Autodesk Inventor part; units mm, degrees
ref_plane "Plano de trabajo4" through (10, 0, 0) normal (1, 0, 0) x (0, 1, 0)
ref_plane "YZ Plane" through (0, 0, 0) normal (1, 0, 0) x (0, 1, 0)
ref_plane "XZ Plane" through (0, 0, 0) normal (0, 1, 0) x (-1, 0, 0)
sketch "Boceto1" plane through (0, 0, 0) normal (0, 0, 1) x (1, 0, 0)
  line L0 (0, 0) -> (20, 0)
  line L1 (20, 0) -> (20, 18.75)
  line L2 (20, 18.75) -> (0, 18.75)
  line L3 (0, 18.75) -> (0, 0)
  point P0 (9.375, 9.375)
  dimension "d0" = 20
  dimension "d10" = 18.75
extrude "Extrusión1" add sketch "Boceto1" against normal blind 56.25
sketch "Boceto2" plane through (0, 0, 0) normal (0, 0, 1) x (1, 0, 0)
  circle A0 centre (10, 9.375) radius 4
  line L0 (0, 0) -> (20, 0)
  line L1 (0, 18.75) -> (0, 0)
  point P0 (10, 0)
  point P1 (0, 9.375)
  dimension "d3" = 8
extrude "Extrusión2" cut sketch "Boceto2" against normal blind 10
fillet "Empalme1" radius 2 4 edges at (20, 0, -28.125) (0, 0, -28.125) (0, 18.75, -28.125) (20, 18.75, -28.125)
sketch "Boceto3" plane through (0, 0, -56.25) normal (0, 0, -1) x (-1, 0, 0)
  line L0 (-20, 16.75) -> (-20, 2)
  line L1 (-18, 0) -> (-2, 0)
  line L2 (-5, 18.75) -> (-15, 18.75)
  line L3 (-15, 18.75) -> (-15, 0)
  line L4 (-15, 0) -> (-5, 0)
  line L5 (-5, 0) -> (-5, 18.75)
  line L6 (-5, 18.75) -> (-15, 0) construction
  line L7 (-15, 18.75) -> (-5, 0) construction
  line L8 (-2, 18.75) -> (-18, 18.75)
  point P0 (0, 0)
  point P1 (-10, 10)
  point P2 (-10, 9.375)
  dimension "d11" = 10
extrude "Extrusión3" cut sketch "Boceto3" against normal blind 10
ref_plane "Plano de trabajo4" through (10, 0, 0) normal (1, 0, 0) x (0, 1, 0)
sketch "Boceto5" plane through (0, 2, 0) normal (-1, 0, 0) x (0, 0, 1)
  circle A0 centre (-28.125, 7) radius 4
  line L0 (0, 14.75) -> (0, 0)
  line L1 (0, 0) -> (-56.25, 0)
  point P0 (0, -2)
  dimension "d20" = 8
  dimension "d21" = 28.125
  dimension "d22" = 7
extrude "Extrusión5" add sketch "Boceto5" along normal blind 10 and the other way blind 30
sketch "Boceto6" plane through (15, 0, -56.25) normal (-1, 0, 0) x (0, 0, 1)
  line L0 (0, 0) -> (56.25, 0)
  line L1 (56.25, 13.375) -> (56.25, 5.375)
  arc A0 (2.5, 12.4975) -> (7.5, 12.4975) centre (5, 9.375) ccw
  line L2 (2.5, 12.4975) -> (7.5, 12.4975)
  line L3 (7.5, 12.4975) -> (7.5, 7.9975)
  line L4 (7.5, 7.9975) -> (2.5, 7.9975)
  line L5 (2.5, 7.9975) -> (2.5, 12.4975)
  dimension "d38" = 8
  dimension "d39" = 9.375
  dimension "d40" = 51.25
  dimension "d41" = 5
  dimension "d42" = 4.5
extrude "Extrusión6" add sketch "Boceto6" along normal up to next contours L5 L4 L3 A0
properties part number "Ante pierna"
Could you check a few things on this model? Use its own coordinates, in mm. A direction names the side the tool comes from. Give positions to 0.01 mm unless a question says otherwise; leave off trailing zeros. Write each loop counter-clockwise with the first axis right and the second up, starting at its lowest first coordinate (ties: lowest second). Pieces come first, ordered by that corner, then holes. Notation, with made-up numbers: (75.5, 48.5) - (88.5, 48.5) arc R25 ccw to (88.5, 87.5) - close; hole circle Ø1 at (5, 84.5). An arc over 180 degrees is marked (long way). One line per item, written item: value. Start each with the question number.
Item 1: If we mould it in two halves opening along X, with no side actions, what happens to faces 6 (the face through (10, 10, -46.25)), 7 (the face through (0, 14, -28)), 8 (the face through (20, 4, -28)), 9 (the face through (6.004, 9.551, -4.93))? For each: +X half, -X half, draft (parallel to the pull), parting line (faces both ways), or undercut.
Item 2: Which directions (+Z, -Z, +X, -X, +Y, -Y) give clear straight access to the entire face, cutting with the end or side of a thin tool? Please do faces 1 (the face through (10, 9, -10)), 2 (the face through (19.4, 18.18, -28.52)), 3 (the face through (10, 10, -48.75)), 4 (the face through (10.07, 5.377, -51.112)), 5 (the face through (-4.93, 11.43, -31.3)).
Item 3: Imagine slicing it at D-D, the plane y = 3. List the corners of the cut face in (x, z) for me.
Item 4: Imagine slicing it at B-B, the plane z = -9. List the corners of the cut face in (x, y) for me (3 decimals).
Item 5: I'm going to push flat-ended pins straight in: pin 1 (2 mm diameter, centred on x = 1, z = -36.5, fed in from -Y); pin 2 (7 mm diameter, centred on x = 10, y = 9.375, fed in from -Z); pin 3 (4 mm diameter, centred on x = 12.5, z = -51.5, fed in from +Y); pin 4 (4 mm diameter, centred on x = -2.5, y = 9, fed in from -Z) (3 decimals). Where does each tip first touch, or does it pass through?
Item 6: Please list where these lines run through material, in increasing order: line 1 (Y direction, x = 10, z = -4) (3 decimals); line 2 (X direction, y = 9.75, z = -51.5); line 3 (X direction, y = 13.5, z = -2.5). Write a range as from..to.
Geometry says:
1. face 6: undercut
1. face 7: -X half
1. face 8: +X half
1. face 9: undercut
2. face 1: +Z
2. face 2: +Z, -Z, +X, +Y
2. face 3: +Y
2. face 4: none
2. face 5: -X
3. outline: (0, -56.25) - (5, -56.25) - (5, -46.25) - (15, -46.25) - (15, -56.25) - (20, -56.25) - (20, 0) - (0, 0) - close
4. outline: (0, 2) arc R2 ccw to (2, 0) - (18, 0) arc R2 ccw to (20, 2) - (20, 16.75) arc R2 ccw to (18, 18.75) - (2, 18.75) arc R2 ccw to (0, 16.75) - close; hole circle Ø8 at (10, 9.375)
5. pin 1: y = 0
5. pin 2: z = -55.25
5. pin 3: y = 8
5. pin 4: z = -32.125
6. line 1: 0..5.375, 13.375..18.75
6. line 2: 0..5, 15..20
6. line 3: 0..20
